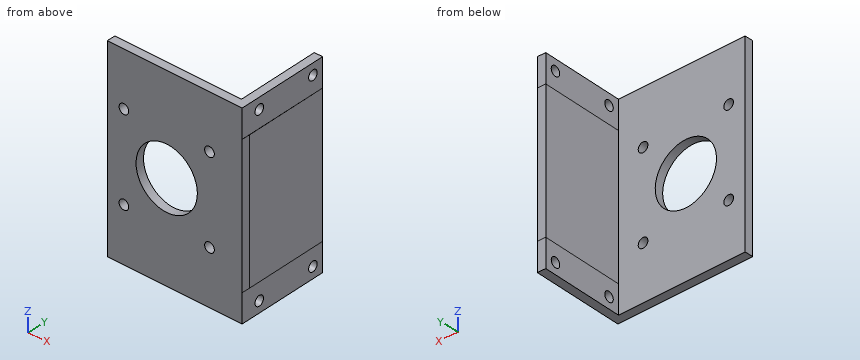
```python
from build123d import *

# Parameters (mm, degrees)
ESBO_O1_R                = 1.75
RESSALTO_EXTRUS_O1_DEPTH = 3
CORTE_EXTRUS_O1_DEPTH    = 70.752508915
ESBO_O6_W                = 3
ESBO_O6_H                = 49.7
RESSALTO_EXTRUS_O2_DEPTH = 30
RESSALTO_EXTRUS_O5_DEPTH = 10.15
RESSALTO_EXTRUS_O6_DEPTH = 10.15
ESBO_O13_R               = 1.75
CORTE_EXTRUS_O2_DEPTH    = 84.696604677
ESBO_O14_R               = 11.1
CORTE_EXTRUS_O3_DEPTH    = 83.873825012


with BuildPart() as part:
    # Esboço1 → Ressalto-extrusão1 (new body)
    with BuildSketch(Plane(origin=(0, 0, 0), x_dir=(1, 0, 0), z_dir=(0, 1, 0))):
        Polygon((0, 0), (0, 49.7), (42, 49.7), (44.85, 49.7), (45.85, 49.7), (48.85, 49.7), (48.85, 0), (44.85, 0), (42, 0), align=None)
        with Locations(Location((6, 9.35, 0), (0, 0, 270))):
            Circle(ESBO_O1_R, mode=Mode.SUBTRACT)
        with Locations(Location((37, 40.35, 0), (0, 0, 270))):
            Circle(ESBO_O1_R, mode=Mode.SUBTRACT)
        with Locations(Location((37, 9.35, 0), (0, 0, 270))):
            Circle(ESBO_O1_R, mode=Mode.SUBTRACT)
        with Locations(Location((6, 40.35, 0), (0, 0, 270))):
            Circle(ESBO_O1_R, mode=Mode.SUBTRACT)
    extrude(amount=RESSALTO_EXTRUS_O1_DEPTH)

    # Esboço4 → Corte-extrusão1 (cut, through all)
    with BuildSketch(Plane.XY):
        Polygon((48.85, 3), (45.850456915, 2.947642781), (45.824605163, 4.428688653), (48.712091154, 4.253252959), (49.11238384, 3.101191082), align=None)
    extrude(amount=-CORTE_EXTRUS_O1_DEPTH, mode=Mode.SUBTRACT)

    # Esboço6 → Ressalto-extrusão2 (add)
    with BuildSketch(Plane(origin=(-0.037470195, 2.146666034, 0), x_dir=(0.9998476951563913, 0.01745240643728361, 0), z_dir=(-0.01745240643728361, 0.9998476951563913, 0))):
        with Locations((47.394917128, 24.85)):
            Rectangle(ESBO_O6_W, ESBO_O6_H)
    extrude(amount=RESSALTO_EXTRUS_O2_DEPTH)

    # Esboço9 → Ressalto-extrusão5 (add)
    with BuildSketch(Plane.XY):
        Polygon((48.326427807, 32.995430855), (48.85, 0), (0, 0), (0, 3), (45.849543016, 3), (45.326884721, 32.943073635), align=None)
    extrude(amount=RESSALTO_EXTRUS_O5_DEPTH)

    # Esboço12 → Ressalto-extrusão6 (add)
    with BuildSketch(Plane(origin=(0, 0, -49.7), x_dir=(-1, 0, 0), z_dir=(0, 0, -1))):
        Polygon((0, 0), (-48.85, 0), (-48.326427807, 32.995430855), (-45.326884721, 32.943073635), (-45.849543016, 3), (0, 3), align=None)
    extrude(amount=RESSALTO_EXTRUS_O6_DEPTH)

    # Esboço13 → Corte-extrusão2 (cut, through all)
    with BuildSketch(Plane(origin=(48.887470195, 0.853333966, 0), x_dir=(0, 0, -1), z_dir=(0.9998476951563913, 0.01745240643728361, 0))):
        with Locations(Location((-6.15, 28.146993031, 0), (0, 0, 90))):
            Circle(ESBO_O13_R)
        with Locations(Location((-6.15, 6.146993031, 0), (0, 0, 90))):
            Circle(ESBO_O13_R)
        with Locations(Location((55.85, 28.146993031, 0), (0, 0, 90))):
            Circle(ESBO_O13_R)
        with Locations(Location((55.85, 6.146993031, 0), (0, 0, 90))):
            Circle(ESBO_O13_R)
    extrude(amount=-CORTE_EXTRUS_O2_DEPTH, mode=Mode.SUBTRACT)

    # Esboço14 → Corte-extrusão3 (cut, through all)
    with BuildSketch(Plane(origin=(0, 3, 0), x_dir=(1, 0, 0), z_dir=(0, 1, 0))):
        with Locations(Location((21.5, 24.85, 0), (0, 0, 270))):
            Circle(ESBO_O14_R)
    extrude(amount=-CORTE_EXTRUS_O3_DEPTH, mode=Mode.SUBTRACT)


solid = part.part
```
Source: CAD feature listing. Evaluate the final solid. Frame: model axes, mm. Coordinates: 2 decimals unless noted, no trailing zeros. Loops run counter-clockwise (first coordinate to the right, second up) from the corner with the lowest first, then second, coordinate; pieces in that order, holes last. Notation, with made-up numbers: (18.5, 85) -> (28.5, 85) arc R28 ccw to (28.5, 103) -> close; hole circle Ø1 at (-23, 69.25). An arc over 180 degrees is marked (long way). One line per item, written item: value. Start each with the question number.
Q1. Contact query for flat-ended pins moving along their axis: P1, Ø3, axis at x = 37, z = -9.35, coming from the -Y side; P2, Ø12, axis at x = 8.5, z = -39.5, coming from the +Y side; P3, Ø4, axis at y = 22.5, z = -7, coming from the -X side. Output: stop coordinate, or through.
Q2. Section query D-D, the plane z = 1. Return the cut outline in (x, y), and give its area (3 significant figures).
Q3. Section query B-B, the plane z = -24.85. Return the cut outline in (x, y).
Q4. Section query C-C, the plane z = -9.35. Return the cut outline in (x, y).
Q5. Section query A-A, the plane x = 21.5. Return the cut outline in (y, z), and give its area (3 significant figures).
Q6. Line query: line 1 along X through (y, z) = (1.55, -40.35); line 2 along X through (y, z) = (1.15, -24.85); line 3 along Y through (x, z) = (30, -52). Output: solid intervals per line, ascending.
Results:
1. P1: through
1. P2: y = 3
1. P3: x = 45.47
2. outline: (0, 0) -> (48.85, 0) -> (48.33, 33) -> (45.33, 32.94) -> (45.85, 3) -> (0, 3) -> close
2. area: 236 mm^2
3. outline: (0, 0) -> (10.4, 0) -> (10.4, 3) -> (0, 3) -> close; (32.6, 0) -> (48.85, 0) -> (48.85, 3) -> (48.33, 33) -> (45.33, 32.94) -> (45.85, 3) -> (32.6, 3) -> close
4. outline: (0, 0) -> (4.25, 0) -> (4.25, 3) -> (0, 3) -> close; (7.75, 0) -> (35.25, 0) -> (35.25, 3) -> (7.75, 3) -> close; (38.75, 0) -> (48.85, 0) -> (48.85, 3) -> (48.33, 33) -> (45.33, 32.94) -> (45.85, 3) -> (38.75, 3) -> close
5. outline: (0, -59.85) -> (3, -59.85) -> (3, -35.95) -> (0, -35.95) -> close; (0, -13.75) -> (3, -13.75) -> (3, 10.15) -> (0, 10.15) -> close
5. area: 143 mm^2
6. line 1: 0 to 4.25, 7.75 to 35.25, 38.75 to 48.85
6. line 2: 0 to 10.4, 32.6 to 48.85
6. line 3: 0 to 3
